from build123d import *

# Parameters (mm, degrees)
SKETCH1_W           = 85.725
SKETCH1_H           = 4.7625
SKETCH1_R           = 1.5875
BOSS_EXTRUDE1_DEPTH = 3.175
BOSS_EXTRUDE2_DEPTH = 4.7625
CUT_EXTRUDE1_REACH  = 38.898
SKETCH3_R           = 1.5875
SKETCH4_W           = 4.7625
SKETCH4_H           = 3.175
BOSS_EXTRUDE3_DEPTH = 25.4
SKETCH5_R           = 1.5875
CUT_EXTRUDE2_DEPTH  = 4.175
SKETCH6_W           = 4.667184745
SKETCH6_H           = 3.175
BOSS_EXTRUDE4_DEPTH = 4.7625


with BuildPart() as part:
    # Sketch1 → Boss-Extrude1 (new body)
    with BuildSketch(Plane(origin=(0, 0, 0), x_dir=(1, 0, 0), z_dir=(0, 1, 0))):
        with Locations((-39.6875, 0)):
            Rectangle(SKETCH1_W, SKETCH1_H)
        Circle(SKETCH1_R, mode=Mode.SUBTRACT)
        with Locations((-79.375, 0)):
            Circle(SKETCH1_R, mode=Mode.SUBTRACT)
    extrude(amount=BOSS_EXTRUDE1_DEPTH)

    # Sketch2 → Boss-Extrude2 (add)
    with BuildSketch(Plane.XY.offset(2.38125)):
        Polygon((-5.58425135, 3.175), (-5.58425135, 6.35), (-26.118044342, 6.35), (-26.118044342, 7.874), (-22.943044342, 7.874), (-22.943044342, 9.144), (-39.512783425, 9.144), (-60.484551788, 30.115768363), (-62.729615818, 27.870704333), (-57.751955743, 22.893044257), (-76.185480906, 4.459519094), (-76.185480906, 3.175), (-72.979871939, 3.175), (-55.506891712, 20.647980227), (-48.771699622, 13.912788136), (-59.509487758, 3.175), (-55.019359697, 3.175), (-46.526635591, 11.667724106), (-38.033911485, 3.175), align=None)
    extrude(amount=-BOSS_EXTRUDE2_DEPTH)

    # Sketch3 → Cut-Extrude1 (cut, up to next)
    with BuildSketch(Plane(origin=(-15.184391712, -15.184391712, 0), x_dir=(0, 0, -1), z_dir=(0.707106781, 0.707106781, 0)), mode=Mode.PRIVATE) as cut_extrude1_sk1:
        with Locations((0, 49.776600757)):
            Circle(SKETCH3_R)
    cut_extrude1_tool1 = extrude(cut_extrude1_sk1.sketch, amount=-CUT_EXTRUDE1_REACH, mode=Mode.PRIVATE) & part.part
    add(cut_extrude1_tool1.solids().sort_by_distance((-50.381764, 20.01298, 0))[0], mode=Mode.SUBTRACT)
    # Sketch3 → Cut-Extrude1 (cut, up to next)
    with BuildSketch(Plane(origin=(-15.184391712, -15.184391712, 0), x_dir=(0, 0, -1), z_dir=(0.707106781, 0.707106781, 0)), mode=Mode.PRIVATE) as cut_extrude1_sk2:
        with Locations((0, 37.076600757)):
            Circle(SKETCH3_R)
    cut_extrude1_tool2 = extrude(cut_extrude1_sk2.sketch, amount=-CUT_EXTRUDE1_REACH, mode=Mode.PRIVATE) & part.part
    add(cut_extrude1_tool2.solids().sort_by_distance((-41.401508, 11.032724, 0))[0], mode=Mode.SUBTRACT)

    # Sketch4 → Boss-Extrude3 (add)
    with BuildSketch(Plane(origin=(3.175, 0, 0), x_dir=(0, 0, -1), z_dir=(1, 0, 0))):
        with Locations((0, 1.5875)):
            Rectangle(SKETCH4_W, SKETCH4_H)
    extrude(amount=BOSS_EXTRUDE3_DEPTH)

    # Sketch5 → Cut-Extrude2 (cut, through all)
    with BuildSketch(Plane(origin=(0, 3.175, 0), x_dir=(1, 0, 0), z_dir=(0, 1, 0))):
        with Locations((12.7, 0)):
            Circle(SKETCH5_R)
        with Locations((25.4, 0)):
            Circle(SKETCH5_R)
    extrude(amount=-CUT_EXTRUDE2_DEPTH, mode=Mode.SUBTRACT)

    # Sketch6 → Boss-Extrude4 (add)
    with BuildSketch(Plane.XY.offset(2.38125)):
        with Locations((19.512903732, 4.7625)):
            Rectangle(SKETCH6_W, SKETCH6_H)
    extrude(amount=-BOSS_EXTRUDE4_DEPTH)


solid = part.part
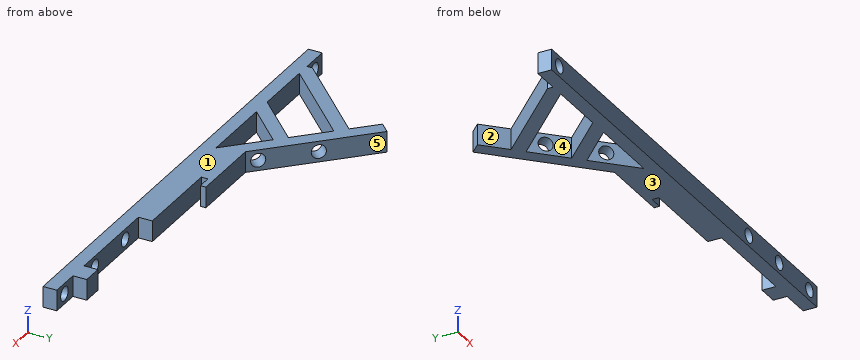
Geometry: final body of the model. Coordinates: model frame, mm. Face numbers are marked on the shaded views. A direction names the side the tool comes from. Round coordinates to 2 decimals unless told otherwise and drop trailing zeros. Loops run counter-clockwise (first coordinate to the right, second up) from the corner with the lowest first, then second, coordinate; pieces in that order, holes last. Notation, with made-up numbers: (53.5, -30.5) -> (85.5, -30.5) arc R25 cw to (85.5, -18.5) -> close; hole circle Ø1 at (24.5, 25). An arc over 180 degrees is marked (long way). One line per question, with ' | ' between items. Start each with the question number.
1. Mould query, pull axis Y, two halves, no side actions, for the marked faces 3, 4 and 5. Classes: pulls with the +Y half, pulls with the -Y half, needs draft (parallel to the pull), parting line crosses it, or undercut.
2. Section C-C on z = 0. Count the separate pieces of the cut face and the enclosed holes in it, and give its area (3 significant figures).
3. Line query: line 1 along Z through (x, y) = (12.7, 2.1); line 2 along X through (y, z) = (3, 0.6) (3 decimals); line 3 along X through (y, z) = (8, 1.7) (3 decimals). Output: solid intervals per line, ascending. Write a range as [from, to].
4. Section B-B on x = -15. Output: boundary loops of the cut face in (y, z).
5. Set-up query: the marked faces 1 and 2. Return all of +Z, -Z, +X, -X, +Y, -Y with unobstructed straight access to the full face (end or side cutting, diameter ignored); none if empty.
6. Section A-A on x = 25.4. Output: boundary loops of the cut face in (y, z) (1 decimal).
7. Section D-D on x = 9. Output: boundary loops of the cut face in (y, z) (3 decimals), and give its area (3 significant figures).
8. Contact query for flat-ended pins moving along their axis: pin 1 (1 mm diameter, centred on x = 3.5, z = -0.5, fed in from +Y) (3 decimals); pin 2 (1.4 mm diameter, centred on x = -63, z = -1, fed in from +Y); pin 3 (2 mm diameter, centred on y = 24, z = -1, fed in from -X). Output: stop coordinate, or through.
Returned:
1) face 3: needs draft | face 4: undercut | face 5: pulls with the +Y half
2) separate pieces: 5 | enclosed holes: 0 | area: 680 mm2
3) line 1: z = [-2.38, -1.59], [1.59, 2.38] | line 2: x = [-82.55, -80.845], [-77.905, -1.47], [1.47, 11.23], [14.17, 23.93], [26.87, 28.575] | line 3: x = [-72.645, -68.155], [-54.684, -50.194], [-42.859, -22.943]
4) outline: (0, -2.38) -> (6.35, -2.38) -> (6.35, 2.38) -> (0, 2.38) -> close
5) face 1: +Z, +X, -X, +Y, -Y | face 2: +Z, -Z, -X
6) outline: (0, -2.4) -> (3.2, -2.4) -> (3.2, -1.6) -> (0, -1.6) -> close; (0, 1.6) -> (3.2, 1.6) -> (3.2, 2.4) -> (0, 2.4) -> close
7) outline: (0, -2.381) -> (3.175, -2.381) -> (3.175, 2.381) -> (0, 2.381) -> close | area: 15.1 mm2
8) pin 1: stops at y = 3.175 | pin 2: stops at y = 28.3 | pin 3: stops at x = -59.86
